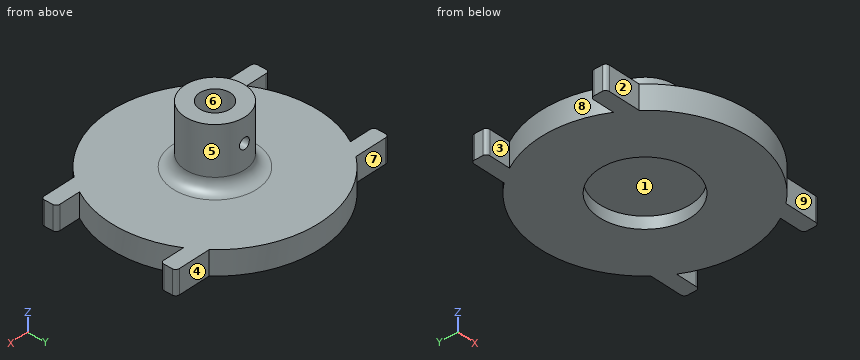
from build123d import *

# Parameters (mm, degrees)
BOSS_EXTRUDE1_DEPTH = 5.08
SKETCH5_R           = 9.6901
CUT_EXTRUDE2_DEPTH  = 2.54
SKETCH6_R           = 6.35
SKETCH6_R_2         = 3.2385
BOSS_EXTRUDE4_DEPTH = 12.7
FILLET1_R           = 2.54
SKETCH8_R           = 1.143
CUT_EXTRUDE3_DEPTH  = 7.62


with BuildPart() as part:
    # Sketch1 → Boss-Extrude1 (new body)
    with BuildSketch(Plane.XY):
        with BuildLine():
            Line((-23.828545778, 14.351), (-16.970545778, 14.351))
            ThreePointArc((-16.970545778, 14.351), (0, 22.225), (16.970545778, 14.351))
            Line((16.970545778, 14.351), (23.828545778, 14.351))
            ThreePointArc((23.828545778, 14.351), (24.367361145, 14.127815367), (24.590545778, 13.589))
            Line((24.590545778, 13.589), (24.590545778, 11.811))
            ThreePointArc((24.590545778, 11.811), (24.367361145, 11.272184633), (23.828545778, 11.049))
            Line((23.828545778, 11.049), (19.283936942, 11.049))
            ThreePointArc((19.283936942, 11.049), (22.225, 0), (19.283936942, -11.049))
            Line((19.283936942, -11.049), (23.828545778, -11.049))
            ThreePointArc((23.828545778, -11.049), (24.367361145, -11.272184633), (24.590545778, -11.811))
            Line((24.590545778, -11.811), (24.590545778, -13.589))
            ThreePointArc((24.590545778, -13.589), (24.367361145, -14.127815367), (23.828545778, -14.351))
            Line((23.828545778, -14.351), (16.970545778, -14.351))
            ThreePointArc((16.970545778, -14.351), (0, -22.225), (-16.970545778, -14.351))
            Line((-16.970545778, -14.351), (-23.828545778, -14.351))
            ThreePointArc((-23.828545778, -14.351), (-24.367361145, -14.127815367), (-24.590545778, -13.589))
            Line((-24.590545778, -13.589), (-24.590545778, -11.811))
            ThreePointArc((-24.590545778, -11.811), (-24.367361145, -11.272184633), (-23.828545778, -11.049))
            Line((-23.828545778, -11.049), (-19.283936942, -11.049))
            ThreePointArc((-19.283936942, -11.049), (-22.225, 0), (-19.283936942, 11.049))
            Line((-19.283936942, 11.049), (-23.828545778, 11.049))
            ThreePointArc((-23.828545778, 11.049), (-24.367361145, 11.272184633), (-24.590545778, 11.811))
            Line((-24.590545778, 11.811), (-24.590545778, 13.589))
            ThreePointArc((-24.590545778, 13.589), (-24.367361145, 14.127815367), (-23.828545778, 14.351))
        make_face()
    extrude(amount=BOSS_EXTRUDE1_DEPTH)

    # Sketch5 → Cut-Extrude2 (cut)
    with BuildSketch(Plane(origin=(0, 0, 0), x_dir=(-1, 0, 0), z_dir=(0, 0, -1))):
        Circle(SKETCH5_R)
    extrude(amount=-CUT_EXTRUDE2_DEPTH, mode=Mode.SUBTRACT)

    # Sketch6 → Boss-Extrude4 (add)
    with BuildSketch(Plane.XY.offset(5.08)):
        Circle(SKETCH6_R)
        Circle(SKETCH6_R_2, mode=Mode.SUBTRACT)
    extrude(amount=BOSS_EXTRUDE4_DEPTH)

    # Fillet1
    fillet1_edges = [part.edges().sort_by_distance(p)[0] for p in [
        (-6.35, 0, 5.08),
    ]]
    fillet(fillet1_edges, radius=FILLET1_R)

    # Sketch8 → Cut-Extrude3 (cut)
    with BuildSketch(Plane(origin=(0, 6.35, 0), x_dir=(1, 0, 0), z_dir=(0, 1, 0))):
        with Locations((0, -12.7)):
            Circle(SKETCH8_R)
    extrude(amount=-CUT_EXTRUDE3_DEPTH, mode=Mode.SUBTRACT)


solid = part.part
Design review of the part built by this model. Coordinates are the model's own, in mm. Face numbers are marked on the shaded views. A direction names the side the tool comes from. Round coordinates to 2 decimals unless told otherwise and drop trailing zeros. Write each loop counter-clockwise with the first axis right and the second up, starting at its lowest first coordinate (ties: lowest second). Pieces come first, ordered by that corner, then holes. Notation, with made-up numbers: (11, -37) - (70, -37) arc R32 cw to (70, -7) - close; hole circle Ø8 at (10, 6). An arc over 180 degrees is marked (long way). Return JSON: item names as keys, results as strings. Group by question number.
Item 1: We need section C-C on x = 21.5. Write out the cut boundary in (y, z).
Item 2: We need section B-B on z = 3.75. Write out the cut boundary in (x, y) (3 decimals), and give its area (3 significant figures).
Item 3: For probe 1 along Y at (x, z) = (0, 14.25); probe 2 along Z at (x, y) = (11.5, -7); probe 3 along X at (y, z) = (4.9, 12.7), list the stretches that pass through material, from the lowest coordinate up. Write a range as [from, to].
Item 4: Machinability: for the marked faces 1, 2, 3, 4 and 5, which of the approach directions +Z, -Z, +X, -X, +Y, -Y give a long, thin tool a straight path to every point of the face, cutting with its end or side? Answer none if there is none.
Item 5: Insertion check: P1, Ø3.5, axis at x = 20.5, z = 3.5, coming from the -Y side; P2, Ø5.5, axis at x = 20, z = 2.5, coming from the +Y side; P3, Ø3, axis at x = -0.5, y = 0, coming from the +Z side; P4, Ø2, axis at y = 8, z = 15, coming from the -X side. Each pin has a flat end and moves straight along its axis. Give the tip position at first contact, or say it passes through.
Item 6: The part is to be moulded in two halves that separate along Y. For the marked faces 6, 7, 8 and 9, say which applies: pulls with the +Y half, pulls with the -Y half, needs draft (parallel to the pull), parting line crosses it, or undercut.
Model answer:
{
 "1": {"outline": "(-14.35, 0) - (-11.05, 0) - (-11.05, 5.08) - (-14.35, 5.08) - close; (-5.63, 0) - (5.63, 0) - (5.63, 5.08) - (-5.63, 5.08) - close; (11.05, 0) - (14.35, 0) - (14.35, 5.08) - (11.05, 5.08) - close"},
 "2": {"outline": "(-24.591, -13.589) arc R0.762 ccw to (-23.829, -14.351) - (-16.971, -14.351) arc R22.225 ccw to (16.971, -14.351) - (23.829, -14.351) arc R0.762 ccw to (24.591, -13.589) - (24.591, -11.811) arc R0.762 ccw to (23.829, -11.049) - (19.284, -11.049) arc R22.225 ccw to (19.284, 11.049) - (23.829, 11.049) arc R0.762 ccw to (24.591, 11.811) - (24.591, 13.589) arc R0.762 ccw to (23.829, 14.351) - (16.971, 14.351) arc R22.225 ccw to (-16.971, 14.351) - (-23.829, 14.351) arc R0.762 ccw to (-24.591, 13.589) - (-24.591, 11.811) arc R0.762 ccw to (-23.829, 11.049) - (-19.284, 11.049) arc R22.225 ccw to (-19.284, -11.049) - (-23.829, -11.049) arc R0.762 ccw to (-24.591, -11.811) - close", "area": "1,640 mm²"},
 "3": {"probe 1": "y = [-6.35, -3.24], [3.24, 6.35]", "probe 2": "z = [0, 5.08]", "probe 3": "x = [-4.04, -1.14], [1.14, 4.04]"},
 "4": {"face 1": "-Z", "face 2": "+Z, -Z, -X, -Y", "face 3": "+Z, -Z, -X", "face 4": "+Z, -Z, +X, +Y", "face 5": "+Z"},
 "5": {"P1": "stops at y = -14.35", "P2": "stops at y = 14.35", "P3": "stops at z = 5.08", "P4": "passes through"},
 "6": {"face 6": "undercut", "face 7": "pulls with the +Y half", "face 8": "undercut", "face 9": "pulls with the -Y half"}
}
